from build123d import *

# Parameters (mm, degrees)
BASE_FLANGE1_START                            = -2
BASE_FLANGE1_DEPTH                            = 2
SKETCH8_R                                     = 1.635
CUT_EXTRUDE1_DEPTH                            = 2
CSK_FOR_4_FLAT_HEAD_SOCKET_CAP_SCREW1_A_COUNT = 2
CSK_FOR_4_FLAT_HEAD_SOCKET_CAP_SCREW1_A_PITCH = 22.95
CUT_EXTRUDE2_DEPTH                            = 2


# Read off the part's stored shape, not the designer's step: Base-Flange1
with BuildPart() as part:
    # Base-Flange1 outline → Base-Flange1 (new body)
    with BuildSketch(Plane(origin=(0, 0, 0), x_dir=(1, 0, 0), z_dir=(0, 1, 0)).offset(BASE_FLANGE1_START)):
        with BuildLine():
            ThreePointArc((-29.187643745, 3.176759435), (-22.95, 7), (-16.712356255, 3.176759435))
            ThreePointArc((-16.712356255, 3.176759435), (-11.475, 1.832537182), (-6.237643745, 3.176759435))
            ThreePointArc((-6.237643745, 3.176759435), (0, 7), (6.237643745, 3.176759435))
            ThreePointArc((6.237643745, 3.176759435), (11.475, 1.832537182), (16.712356255, 3.176759435))
            ThreePointArc((16.712356255, 3.176759435), (22.95, 7), (29.187643745, 3.176759435))
            Line((29.187643745, 3.176759435), (29.187643745, 25.875))
            Line((29.187643745, 25.875), (-19.187643745, 25.875))
            Line((-19.187643745, 25.875), (-19.187643745, 48.375))
            Line((-19.187643745, 48.375), (-29.187643745, 48.375))
            Line((-29.187643745, 48.375), (-29.187643745, 3.176759435))
        make_face()
    extrude(amount=BASE_FLANGE1_DEPTH)

    # Sketch8 → Cut-Extrude1 (cut)
    with BuildSketch(Plane(origin=(0, 0, 0), x_dir=(1, 0, 0), z_dir=(0, 1, 0))):
        with Locations(Location((-24.187643745, 44.375, 0), (0, 0, 270))):
            Circle(SKETCH8_R)
        with Locations(Location((-24.187643745, 34.875, 0), (0, 0, 270))):
            Circle(SKETCH8_R)
    extrude(amount=-CUT_EXTRUDE1_DEPTH, mode=Mode.SUBTRACT)

    # Sketch10 → CSK for #4 Flat Head Socket Cap Screw1 (revolve, cut)
    with BuildSketch(Plane(origin=(11.475, 0, -18.375), x_dir=(0, 0, 1), z_dir=(1, 0, 0))):
        Polygon((0, 0), (0, 2.980574487), (1.63195, 2), (1.63195, 1.848124365), (3.2385, 0), align=None)
    csk_for_4_flat_head_socket_cap_screw1 = revolve(axis=Axis((11.475, 6.35, -18.375), (0, -1, 0)), mode=Mode.SUBTRACT)

    # CSK for #4 Flat Head Socket Cap Screw1 a: CSK for #4 Flat Head Socket Cap Screw1 ×2
    with Locations(*[(-i * CSK_FOR_4_FLAT_HEAD_SOCKET_CAP_SCREW1_A_PITCH, 0, 0) for i in range(1, CSK_FOR_4_FLAT_HEAD_SOCKET_CAP_SCREW1_A_COUNT)]):
        add(csk_for_4_flat_head_socket_cap_screw1, mode=Mode.SUBTRACT)

    # Sketch12 → Cut-Extrude2 (cut)
    with BuildSketch(Plane(origin=(0, 0, 0), x_dir=(1, 0, 0), z_dir=(0, 1, 0))):
        with BuildLine():
            Line((-29.633189727, 3.403670823), (-29.633189727, -1.121913875))
            Line((-29.633189727, -1.121913875), (35.30589457, -1.121913875))
            Line((35.30589457, -1.121913875), (35.30589457, 25.875))
            Line((35.30589457, 25.875), (28.687643745, 25.875))
            Line((28.687643745, 25.875), (28.687643745, 4.83005634))
            ThreePointArc((28.687643745, 4.83005634), (22.173017349, 7.459644627), (16.340134062, 3.543962794))
            ThreePointArc((16.340134062, 3.543962794), (11.475, 2.332537182), (6.609865938, 3.543962794))
            ThreePointArc((6.609865938, 3.543962794), (0, 7.5), (-6.609865938, 3.543962794))
            ThreePointArc((-6.609865938, 3.543962794), (-11.475, 2.332537182), (-16.340134062, 3.543962794))
            ThreePointArc((-16.340134062, 3.543962794), (-23.029148934, 7.499582351), (-29.633189727, 3.403670823))
        make_face()
    extrude(amount=-CUT_EXTRUDE2_DEPTH, mode=Mode.SUBTRACT)


solid = part.part
For this review, take the finished solid that the model builds, in its own axes (mm). A direction names the side the tool comes from. Coordinates: 2 decimals unless noted, no trailing zeros. Order: outer loops, then holes, each group sorted by start corner. A loop starts at its lowest first (then second) coordinate and runs counter-clockwise, first axis right, second up. Notation, with made-up numbers: (22, -11) - (32, -11) arc R8 cw to (32, 1) - close; hole circle Ø3 at (35, 62.25). An arc over 180 degrees is marked (long way). Answer as CSV lines item,"result". Start each with the question number.
1) Insertion check: P1, Ø4, axis at x = 11.475, z = -18.375, coming from the +Y side; P2, Ø1, axis at x = 9.5, y = -1.5, coming from the -Z side (3 decimals). Each pin has a flat end and moves straight along its axis. Give the tip position at first contact, or say it passes through.
2) To check wall thickness, follow line 1 along X through (y, z) = (-1.45, -18); line 2 along X through (y, z) = (-0.9, -17); line 3 along Z through (x, y) = (-26.5, -1.55) (3 decimals). State the ranges of each line that lie inside material, in increasing order. Write a range as [from, to].
3) Add section C-C (z = -44). State the section outline as (x, y) points, then the cut area to 3 significant figures.
4) Add section B-B (y = -0.3). State the section outline as (x, z) points (3 decimals).
5) Draft analysis for pull direction X (two halves, no side actions). For faces 3 (the flat face through (-24, -1, -48.375)), 4 (the flat face through (-29.188, -1, -27)), 5 (the cylindrical face through (-22.809, -0.986, -33.996)), state which applies: +X half, -X half, draft (parallel to the pull), parting line (faces both ways), or undercut.
6) Machinability: for faces 1 (the cylindrical face through (-11.404, -0.986, -2.333)), 2 (the flat face through (-19.188, -1, -37)), which of the approach directions +Z, -Z, +X, -X, +Y, -Y give a long, thin tool a straight path to every point of the face, cutting with its end or side? Answer none if there is none.
7) Add section A-A (z = -6.5). State the section outline as (x, y) points.
8) Add section D-D (x = -4.5). State the section outline as (y, z) points (3 decimals), then the cut area to 4 significant figures.
Result:
1,P1,"y = -1.42"
1,P2,"z = -25.875"
2,line 1,"[-29.19, -13.42], [-9.53, 9.53], [13.42, 28.69]"
2,line 2,"[-29.19, -13.51], [-9.44, 9.44], [13.51, 28.69]"
2,line 3,"[-48.375, -6.607]"
3,outline,"(-29.19, -2) - (-25.78, -2) - (-25.78, 0) - (-29.19, 0) - close; (-22.6, -2) - (-19.19, -2) - (-19.19, 0) - (-22.6, 0) - close"
3,area,"13.6 mm^2"
4,outline,"(-29.188, -48.375) - (-19.188, -48.375) - (-19.188, -25.875) - (28.688, -25.875) - (28.688, -4.83) arc R7.5 cw to (16.34, -3.544) arc R10.375 ccw to (6.61, -3.544) arc R7.5 cw to (-6.61, -3.544) arc R10.375 ccw to (-16.34, -3.544) arc R7.5 cw to (-29.188, -4.164) - close; hole circle Ø3.27 at (-24.188, -44.375); hole circle Ø3.27 at (-24.188, -34.875); hole circle Ø5.955 at (-11.475, -18.375); hole circle Ø5.955 at (11.475, -18.375)"
5,face 3,"draft"
5,face 4,"-X half"
5,face 5,"undercut"
6,face 1,"+Z, +Y, -Y"
6,face 2,"-Z, +X, +Y, -Y"
7,outline,"(-29.19, -2) - (-26.69, -2) - (-26.69, 0) - (-29.19, 0) - close; (-19.21, -2) - (-3.74, -2) - (-3.74, 0) - (-19.21, 0) - close; (3.74, -2) - (19.21, -2) - (19.21, 0) - (3.74, 0) - close; (26.69, -2) - (28.69, -2) - (28.69, 0) - (26.69, 0) - close"
8,outline,"(-2, -25.875) - (0, -25.875) - (0, -6) - (-2, -6) - close"
8,area,"39.75 mm^2"
